Can you work these out from the drawing? Everything is in mm from the part's minimum corner. A direction names the side the tool comes from. Coordinates: 2 decimals unless noted, no trailing zeros. Order: outer loops, then holes, each group sorted by start corner. A loop starts at its lowest first (then second) coordinate and runs counter-clockwise, first axis right, second up. Notation, with made-up numbers: (6, -40) - (25, -40) arc R16 ccw to (25, -20) - close; hole circle Ø1 at (79, 7.5). An arc over 180 degrees is marked (long way). Answer as CSV lines item,"result". Start each with the question number.
Q1. I need wall thicknesses on line 1 (X direction, y = 109, z = 16.5); line 2 (Y direction, x = 175, z = 27); line 3 (X direction, y = 99, z = 32). Which ranges of each line are inside material? Lowest first, please.
Q2. Suppose I cut it at B-B (z = 8). Please give me the cut outline in (x, y), then the cut area to 3 significant figures.
Q3. Thinking about a two-plate mould opening in X: for the marked faces 3, 4, 5 and 6, which applies, released by +X, released by -X, zero draft, split by the parting line, or undercut?
Q4. Suppose I cut it at A-A (x = 175). Please give me the cut outline in (y, z).
Q5. Suppose I cut it at D-D (x = 320). Please give me the cut outline in (y, z).
Q6. Suppose I cut it at C-C (x = 55). Please give me the cut outline in (y, z).
Q7. For the marked faces 1 and 2, which set-ups out of +Z, -Z, +X, -X, +Y, -Y let a thin tool reach every point of the face, with its end or its side?
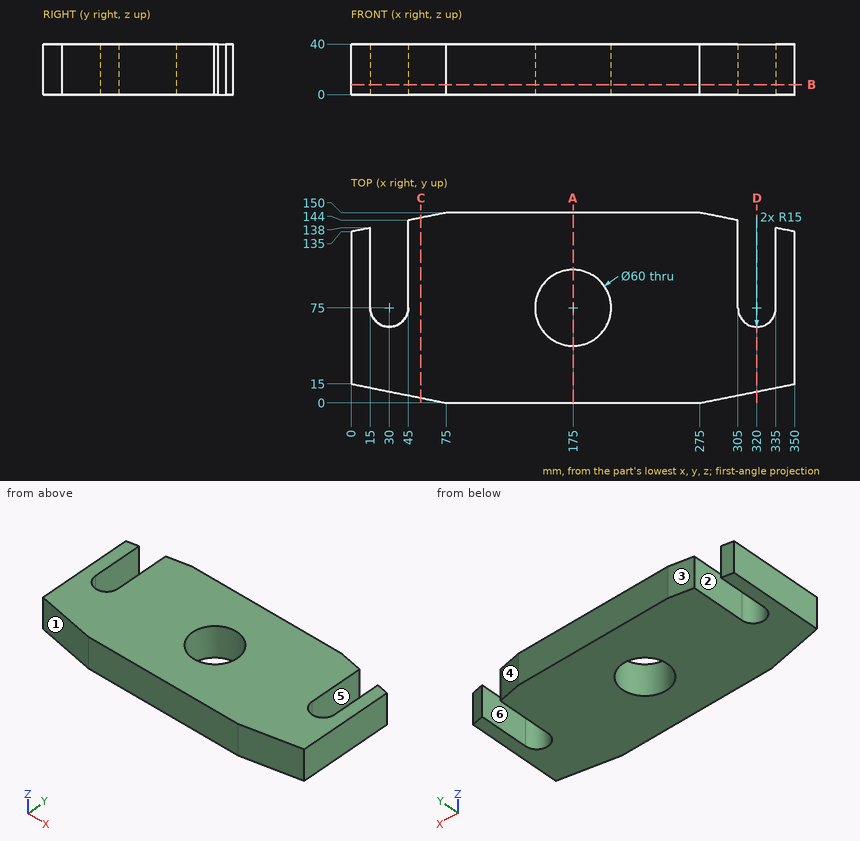
Here are the results:
1,line 1,"x = 0 to 15, 45 to 305, 335 to 350"
1,line 2,"y = 0 to 45, 105 to 150"
1,line 3,"x = 0 to 15, 45 to 157, 193 to 305, 335 to 350"
2,outline,"(0, 15) - (75, 0) - (275, 0) - (350, 15) - (350, 135) - (335, 138) - (335, 75) arc R15 cw to (305, 75) - (305, 144) - (275, 150) - (75, 150) - (45, 144) - (45, 75) arc R15 cw to (15, 75) - (15, 138) - (0, 135) - close; hole circle Ø60 at (175, 75)"
2,area,"42,800 mm²"
3,face 3,"released by -X"
3,face 4,"released by +X"
3,face 5,"undercut"
3,face 6,"undercut"
4,outline,"(0, 0) - (45, 0) - (45, 40) - (0, 40) - close; (105, 0) - (150, 0) - (150, 40) - (105, 40) - close"
5,outline,"(9, 0) - (60, 0) - (60, 40) - (9, 40) - close"
6,outline,"(4, 0) - (146, 0) - (146, 40) - (4, 40) - close"
7,face 1,"+Z, -Z, -X, -Y"
7,face 2,"+Z, -Z, +Y"
